Input: part model. Units: mm. Frame: model coordinates. Face numbers are marked on the shaded views. A direction names the side the tool comes from. Round coordinates to 2 decimals unless told otherwise and drop trailing zeros. Loops run counter-clockwise (first coordinate to the right, second up) from the corner with the lowest first, then second, coordinate; pieces in that order, holes last. Notation, with made-up numbers: (4.5, -20.5) - (46.5, -20.5) arc R30 cw to (46.5, 13.5) - close; hole circle Ø11 at (34, -38). An arc over 180 degrees is marked (long way). One line per question, with ' | ' between items. Start each with the question number.
Item 1: Material intervals for line 1 along X through (y, z) = (1, -5); line 2 along Z through (x, y) = (41, 21); line 3 along Z through (x, y) = (203.5, 0.5), sorted ascending.
Item 2: Section B-B, the plane y = 5.5. Return loops of the section in (x, z).
Item 3: First-contact query: pin 1 (1.3 mm diameter, centred on x = 492.5, y = -21.5, fed in from -Z); pin 2 (3 mm diameter, centred on x = 393.5, z = 4.5, fed in from -Y); pin 3 (12 mm diameter, centred on x = 373.5, z = -2.5, fed in from +Y). Flat tips, straight axial feed; report the tip coordinate or a pass-through.
Item 4: Set-up query: the marked faces 1 and 2. Return all of +Z, -Z, +X, -X, +Y, -Y with unobstructed straight access to the full face (end or side cutting, diameter ignored); none if empty.
Item 5: Draft query along X for the marked faces 3, 4 and 5. Return one class per face: pulls with the +X half, pulls with the -X half, needs draft (parallel to the pull), parting line crosses it, or undercut.
Item 6: Section A-A, the plane z = -9.5. Return loops of the section in (x, y).
Item 7: Section C-C, the plane x = 202.5. Return loops of the section in (y, z), plus the area to 3 significant figures.
```python
from build123d import *

# Parameters (mm, degrees)
BOSS_EXTRUDE5_DEPTH = 30
BOSS_EXTRUDE6_DEPTH = 10


with BuildPart() as part:
    # Sketch1 → Boss-Extrude5 (new, symmetric)
    with BuildSketch(Plane(origin=(0, 0, 0), x_dir=(1, 0, 0), z_dir=(0, 1, 0))):
        with BuildLine():
            Line((245, 0), (236, 0))
            ThreePointArc((236, 0), (227.438690983, -10.319470785), (215.715909091, -3.810717135))
            ThreePointArc((215.715909091, -3.810717135), (215.25, -3.492179856), (214.784090909, -3.810717135))
            ThreePointArc((214.784090909, -3.810717135), (205, -10.5), (195.215909091, -3.810717135))
            ThreePointArc((195.215909091, -3.810717135), (194.75, -3.492179856), (194.284090909, -3.810717135))
            ThreePointArc((194.284090909, -3.810717135), (184.5, -10.5), (174.715909091, -3.810717135))
            ThreePointArc((174.715909091, -3.810717135), (174.25, -3.492179856), (173.784090909, -3.810717135))
            ThreePointArc((173.784090909, -3.810717135), (164, -10.5), (154.215909091, -3.810717135))
            ThreePointArc((154.215909091, -3.810717135), (153.75, -3.492179856), (153.284090909, -3.810717135))
            ThreePointArc((153.284090909, -3.810717135), (143.5, -10.5), (133.715909091, -3.810717135))
            ThreePointArc((133.715909091, -3.810717135), (133.25, -3.492179856), (132.784090909, -3.810717135))
            ThreePointArc((132.784090909, -3.810717135), (123, -10.5), (113.215909091, -3.810717135))
            ThreePointArc((113.215909091, -3.810717135), (112.75, -3.492179856), (112.284090909, -3.810717135))
            ThreePointArc((112.284090909, -3.810717135), (102.5, -10.5), (92.715909091, -3.810717135))
            ThreePointArc((92.715909091, -3.810717135), (92.25, -3.492179856), (91.784090909, -3.810717135))
            ThreePointArc((91.784090909, -3.810717135), (82, -10.5), (72.215909091, -3.810717135))
            ThreePointArc((72.215909091, -3.810717135), (71.75, -3.492179856), (71.284090909, -3.810717135))
            ThreePointArc((71.284090909, -3.810717135), (61.5, -10.5), (51.715909091, -3.810717135))
            ThreePointArc((51.715909091, -3.810717135), (51.25, -3.492179856), (50.784090909, -3.810717135))
            ThreePointArc((50.784090909, -3.810717135), (41, -10.5), (31.215909091, -3.810717135))
            ThreePointArc((31.215909091, -3.810717135), (30.75, -3.492179856), (30.284090909, -3.810717135))
            ThreePointArc((30.284090909, -3.810717135), (20.5, -10.5), (10.715909091, -3.810717135))
            ThreePointArc((10.715909091, -3.810717135), (10.25, -3.492179856), (9.784090909, -3.810717135))
            ThreePointArc((9.784090909, -3.810717135), (-1.938690983, -10.319470785), (-10.5, 0))
            Line((-10.5, 0), (-15, 0))
            Line((-15, 0), (-15, -15))
            Line((-15, -15), (496, -15))
            Line((496, -15), (496, 0))
            Line((496, 0), (491.5, 0))
            ThreePointArc((491.5, 0), (482.938690983, -10.319470785), (471.215909091, -3.810717135))
            ThreePointArc((471.215909091, -3.810717135), (470.75, -3.492179856), (470.284090909, -3.810717135))
            ThreePointArc((470.284090909, -3.810717135), (460.5, -10.5), (450.715909091, -3.810717135))
            ThreePointArc((450.715909091, -3.810717135), (450.25, -3.492179856), (449.784090909, -3.810717135))
            ThreePointArc((449.784090909, -3.810717135), (440, -10.5), (430.215909091, -3.810717135))
            ThreePointArc((430.215909091, -3.810717135), (429.75, -3.492179856), (429.284090909, -3.810717135))
            ThreePointArc((429.284090909, -3.810717135), (419.5, -10.5), (409.715909091, -3.810717135))
            ThreePointArc((409.715909091, -3.810717135), (409.25, -3.492179856), (408.784090909, -3.810717135))
            ThreePointArc((408.784090909, -3.810717135), (399, -10.5), (389.215909091, -3.810717135))
            ThreePointArc((389.215909091, -3.810717135), (388.75, -3.492179856), (388.284090909, -3.810717135))
            ThreePointArc((388.284090909, -3.810717135), (378.5, -10.5), (368.715909091, -3.810717135))
            ThreePointArc((368.715909091, -3.810717135), (368.25, -3.492179856), (367.784090909, -3.810717135))
            ThreePointArc((367.784090909, -3.810717135), (358, -10.5), (348.215909091, -3.810717135))
            ThreePointArc((348.215909091, -3.810717135), (347.75, -3.492179856), (347.284090909, -3.810717135))
            ThreePointArc((347.284090909, -3.810717135), (337.5, -10.5), (327.715909091, -3.810717135))
            ThreePointArc((327.715909091, -3.810717135), (327.25, -3.492179856), (326.784090909, -3.810717135))
            ThreePointArc((326.784090909, -3.810717135), (317, -10.5), (307.215909091, -3.810717135))
            ThreePointArc((307.215909091, -3.810717135), (306.75, -3.492179856), (306.284090909, -3.810717135))
            ThreePointArc((306.284090909, -3.810717135), (296.5, -10.5), (286.715909091, -3.810717135))
            ThreePointArc((286.715909091, -3.810717135), (286.25, -3.492179856), (285.784090909, -3.810717135))
            ThreePointArc((285.784090909, -3.810717135), (276, -10.5), (266.215909091, -3.810717135))
            ThreePointArc((266.215909091, -3.810717135), (265.75, -3.492179856), (265.284090909, -3.810717135))
            ThreePointArc((265.284090909, -3.810717135), (253.561309017, -10.319470785), (245, 0))
        make_face()
    extrude(amount=BOSS_EXTRUDE5_DEPTH, both=True)

    # Sketch6 → Boss-Extrude6 (add, symmetric)
    with BuildSketch(Plane(origin=(0, 0, 0), x_dir=(1, 0, 0), z_dir=(0, 1, 0))):
        Polygon((-15, -15), (496, -15), (496, 15), (470.5, 15), (470.5, 0), (266, 0), (266, 15), (215, 15), (215, 0), (10.5, 0), (10.5, 15), (-15, 15), align=None)
    extrude(amount=BOSS_EXTRUDE6_DEPTH, both=True)


solid = part.part
```
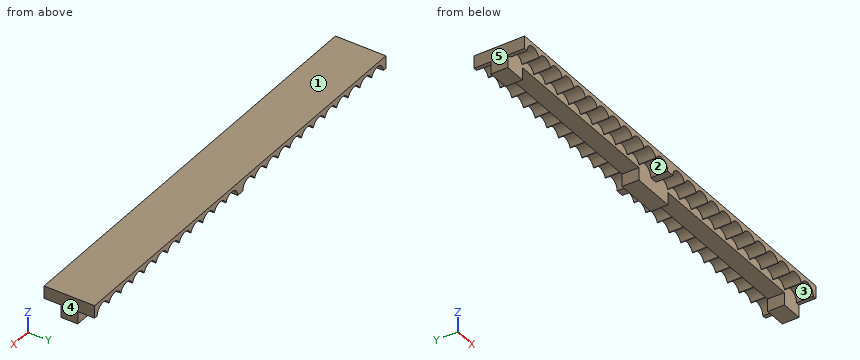
Return value:
1) line 1: -15 to 10.5, 215 to 266, 470.5 to 496 | line 2: 10.5 to 15 | line 3: 0 to 15
2) outline: (-15, -15) - (10.5, -15) - (10.5, 0) - (215, 0) - (215, -15) - (266, -15) - (266, 0) - (470.5, 0) - (470.5, -15) - (496, -15) - (496, 15) - (-15, 15) - close
3) pin 1: z = 0 | pin 2: y = -10 | pin 3: y = 10
4) face 1: +Z, +X, -X, +Y, -Y | face 2: -Z, -Y
5) face 3: undercut | face 4: pulls with the +X half | face 5: pulls with the -X half
6) outline: (-15, -10) - (10.5, -10) - (10.5, 10) - (-15, 10) - close; (215, -10) - (266, -10) - (266, 10) - (215, 10) - close; (470.5, -10) - (496, -10) - (496, 10) - (470.5, 10) - close
7) outline: (-30, 10.2) - (-10, 10.2) - (-10, 0) - (10, 0) - (10, 10.2) - (30, 10.2) - (30, 15) - (-30, 15) - close | area: 492 mm2
